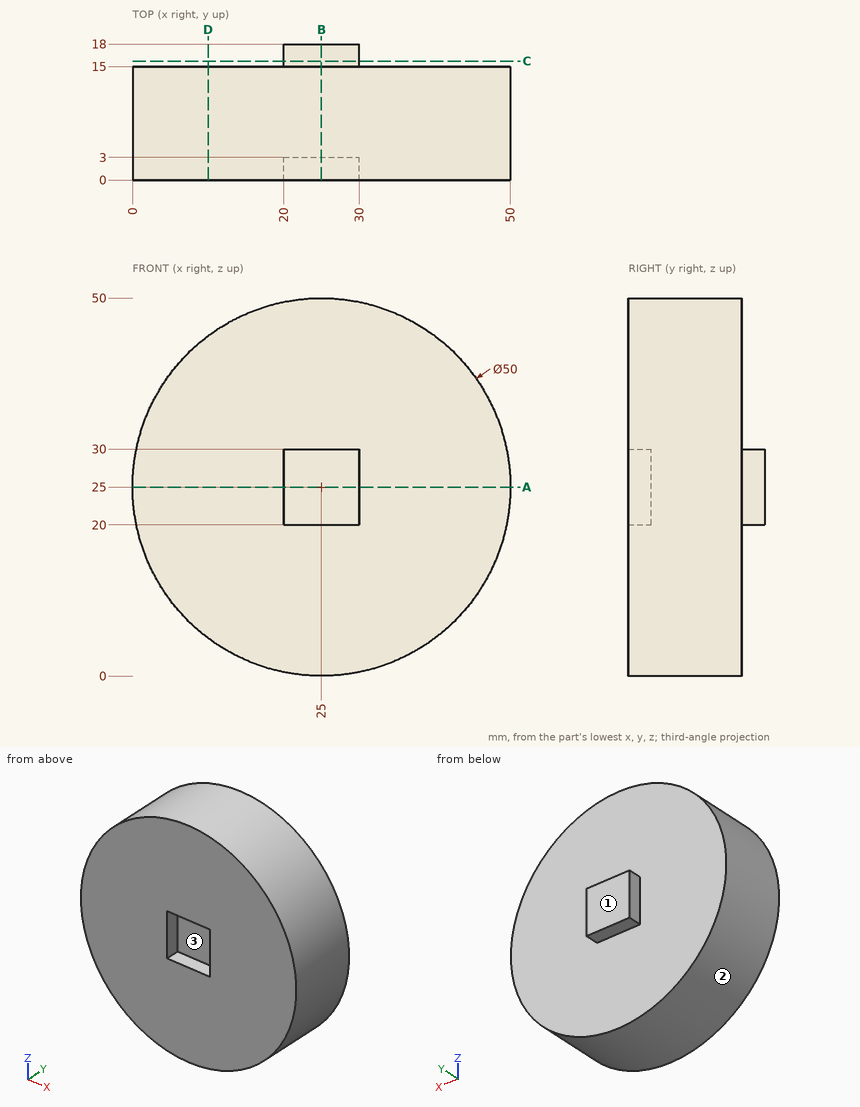
Answer from the drawing. Dimensions are ordinates in mm from the lowest x, y and z of the part. Round coordinates to 2 decimals unless told otherwise and drop trailing zeros. Order: outer loops, then holes, each group sorted by start corner. A loop starts at its lowest first (then second) coordinate and runs counter-clockwise, first axis right, second up.
1) Straight lines are drawn through the part: L1, parallel to Y at x = 25.5, z = 30.5; L2, parallel to X at y = 13.5, z = 25.5 (3 decimals); L3, parallel to X at y = 0.75, z = 27. For each, find the intervals that lie inside material, in ascending order.
2) The part is cut by section D-D on x = 10. Write down the section's boundary in (y, z), plus the area to 3 significant figures.
3) The part is cut by section C-C on y = 15.75. Write down the section's boundary in (x, z), plus the area to 3 significant figures.
4) The part is cut by section B-B on x = 25. Write down the section's boundary in (y, z), plus the area to 3 significant figures.
5) The mould has two halves that part along Z. Classify the marked faces 1, 2 and 3: released by +Z, released by -Z, zero draft, split by the parting line, or undercut.
6) Flat-ended cylindrical pins translate along their axes: pin 1 (1.5 mm diameter, centred on x = 25.5, y = 2, fed in from -Z); pin 2 (0.9 mm diameter, centred on y = 16.5, z = 26, fed in from -X); pin 3 (0.9 mm diameter, centred on x = 23, y = 16, fed in from +Z); pin 4 (1.5 mm diameter, centred on y = 8, z = 39.5, fed in from +X). Find the tip coordinate at first contact, or state that the pin passes through.
7) The part is cut by section A-A on z = 25. Write down the section's boundary in (x, y), plus the area to 3 significant figures.
Resolved:
1. L1: y = 0 to 15
1. L2: x = 0.005 to 49.995
1. L3: x = 0.08 to 20, 30 to 49.92
2. outline: (0, 5) - (15, 5) - (15, 45) - (0, 45) - close
2. area: 600 mm2
3. outline: (20, 20) - (30, 20) - (30, 30) - (20, 30) - close
3. area: 100 mm2
4. outline: (0, 0) - (15, 0) - (15, 20) - (18, 20) - (18, 30) - (15, 30) - (15, 50) - (0, 50) - (0, 30) - (3, 30) - (3, 20) - (0, 20) - close
4. area: 750 mm2
5. face 1: zero draft
5. face 2: split by the parting line
5. face 3: undercut
6. pin 1: stops at z = 0
6. pin 2: stops at x = 20
6. pin 3: stops at z = 30
6. pin 4: stops at x = 45.88
7. outline: (0, 0) - (20, 0) - (20, 3) - (30, 3) - (30, 0) - (50, 0) - (50, 15) - (30, 15) - (30, 18) - (20, 18) - (20, 15) - (0, 15) - close
7. area: 750 mm2
